Source: three-view drawing plus pictorial views. Frame: mm from the lowest corner of the part. A direction names the side the tool comes from. Give positions to 0.01 mm unless a question says otherwise; leave off trailing zeros. Order: outer loops, then holes, each group sorted by start corner. A loop starts at its lowest first (then second) coordinate and runs counter-clockwise, first axis right, second up. Notation, with made-up numbers: (44.5, 17) -> (80.5, 17) arc R22 cw to (80.5, 55) -> close; hole circle Ø5 at (52, -29). An arc over 180 degrees is marked (long way). Write item = value, one per line.
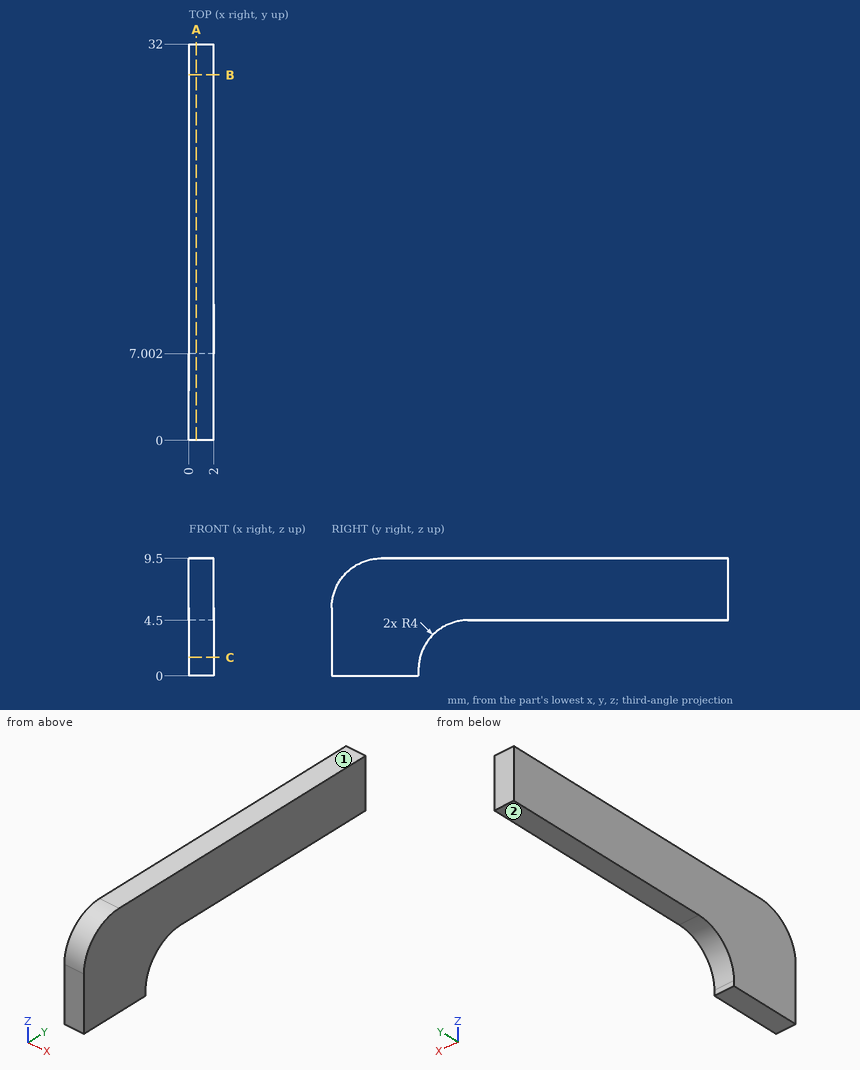
1) Line query: line 1 (Z direction, x = 1.15, y = 21); line 2 (Y direction, x = 0.6, z = 4); line 3 (Y direction, x = 0.25, z = 8.5). Output: solid intervals per line, ascending. Write a range as from..to.
Check sheet entries:
line_1 = 4.5..9.5
line_2 = 0..9.07
line_3 = 1.35..32
2) First-contact query: P1, Ø1, axis at x = 0.5, y = 10.5, coming from the -Z side; P2, Ø1, axis at x = 1, y = 22.5, coming from the -Z side. Flat tips, straight axial feed; report the tip coordinate or a pass-through.
Check sheet entries:
P1 = 4.37
P2 = 4.5
3) Section query C-C (z = 1.5). Output: boundary loops of the cut face in (x, y), plus the area to 3 significant figures.
Check sheet entries:
outline = (0, 0) -> (2, 0) -> (2, 7.13) -> (0, 7.13) -> close
area = 14.3 mm²
4) Section query A-A (x = 0.6). Output: boundary loops of the cut face in (y, z).
Check sheet entries:
outline = (0, 0) -> (7, 0) -> (7, 0.5) arc R4 cw to (11, 4.5) -> (32, 4.5) -> (32, 9.5) -> (4, 9.5) arc R4 ccw to (0, 5.5) -> close
5) Section query B-B (y = 29.5). Output: boundary loops of the cut face in (x, z), plus the area to 3 significant figures.
Check sheet entries:
outline = (0, 4.5) -> (2, 4.5) -> (2, 9.5) -> (0, 9.5) -> close
area = 10.0 mm²
6) Reachability of the marked faces 1 and 2 from +Z, -Z, +X, -X, +Y, -Y: full face, straight path, thin tool, end or side. Return the list, or none.
Check sheet entries:
face_1 = +Z, +X, -X, +Y, -Y
face_2 = -Z, +X, -X, +Y
